Design review of the part built by this model. Coordinates are the model's own, in mm. A direction names the side the tool comes from. Round coordinates to 2 decimals unless told otherwise and drop trailing zeros. Loops run counter-clockwise (first coordinate to the right, second up) from the corner with the lowest first, then second, coordinate; pieces in that order, holes last. Notation, with made-up numbers: (59.25, 65.5) -> (93.25, 65.5) arc R22 ccw to (93.25, 84.5) -> close; hole circle Ø11 at (-40, -8). An arc over 180 degrees is marked (long way). Answer as CSV lines item,"result". Start each with the question number.
(1) Draft analysis for pull direction X (two halves, no side actions). For faces 4 (the face through (-19.15, -107.74, 0.64)), 5 (the face through (-75.61, 27.47, 0.63)), 6 (the face through (-34.96, -102.51, 0.63)), state which applies: +X half, -X half, draft (parallel to the pull), parting line (faces both ways), or undercut.
(2) Take a section at C-C, the plane y = -41. Write out the cut boundary in (x, z) (3 decimals), and give its area (3 significant figures).
(3) Take a section at D-D, the plane x = -88. Write out the cut boundary in (y, z), and give its area (3 significant figures).
(4) Take a section at A-A, the plane x = -77.55. Write out the cut boundary in (y, z).
(5) To check wall thickness, follow line 1 (Y direction, x = -87.55, z = 1); line 2 (Y direction, x = -77.55, z = 0.85); line 3 (X direction, y = -92.5, z = 0.2). State the ranges of each line that lie inside material, in increasing order. Write a range as from..to.
(6) Machinability: for faces 1 (the face through (-59.822, -63.878, 0.644)), 2 (the face through (-41.71, -87.56, 0.63)), 3 (the face through (-93.551, 30.795, 0.644)), which of the approach directions +Z, -Z, +X, -X, +Y, -Y give a long, thin tool a straight path to every point of the face, cutting with its end or side? Answer none if there is none.
(7) Take a section at B-B, the plane z = 0.3. State how many separate pieces and enclosed holes the cut face has, and give its area (3 significant figures).
(8) For P1, Ø4, axis at x = -87.55, y = 28.273, coming from the -Z side; P2, Ø6.5, axis at x = -87.55, y = -20.327, coming from the +Z side; P3, Ø0.6, axis at y = 11.5, z = 0.5, coming from the -X side, all flat-tipped, find the tip position at first contact; note any pin that passes through.
from build123d import *

# Parameters (mm, degrees)
SKETCH1_R                    = 2.099999991
BASE_FLANGE1_DEPTH           = 1.27
EDGE_FLANGE2_STRIP_W         = 6.5532
EDGE_FLANGE2_STRIP_H         = 1.27
EDGE_FLANGE2_STRIP_CUT_DEPTH = 59.775021713
EDGE_FLANGE2_DEPTH           = 59.775021713
SKETCH14_W                   = 1.779250061
SKETCH14_H                   = 41.153999988
CUT_EXTRUDE1_DEPTH           = 148.532360138
CUT_EXTRUDE_THIN2_START      = 2.868175785
CUT_EXTRUDE_THIN2_DEPTH      = 59.775021713
CUT_EXTRUDE_THIN2_START_2    = 9.218175785
CUT_EXTRUDE_THIN2_2_DEPTH    = 47.075021713
CUT_EXTRUDE_THIN2_3_DEPTH    = 59.775021713
CUT_EXTRUDE_THIN2_4_DEPTH    = 6.35
CUT_EXTRUDE_THIN2_START_3    = 56.293197498
CUT_EXTRUDE_THIN2_5_DEPTH    = 6.35
BOSS_EXTRUDE1_DEPTH          = 1.27
FILLET1_R                    = 25.4
FILLET2_R                    = 3.175


# Read off the part's stored shape, not the designer's step: Cut-Extrude-Thin2
# Sheet-metal steps are written as plain solids
with BuildPart() as part:
    # Sketch1 → Base-Flange1 (new body)
    with BuildSketch(Plane.XY):
        Polygon((-24.438645943, -113.029505435), (-19.05049227, -107.641351762), (-63.562879499, -63.128964533), (-66.675, -51.514372705), (-66.675, 31.75), (-94.45625, 31.75), (-94.45625, -51.514372705), (-80.565625, -65.404997705), (-68.951033172, -68.517118206), align=None)
        with Locations((-87.550000033, 28.272999969)):
            Circle(SKETCH1_R, mode=Mode.SUBTRACT)
        with Locations((-77.549999967, 28.272999969)):
            Circle(SKETCH1_R, mode=Mode.SUBTRACT)
        with Locations((-87.550000033, -20.327000113)):
            Circle(SKETCH1_R, mode=Mode.SUBTRACT)
        with Locations((-77.549999967, -20.327000113)):
            Circle(SKETCH1_R, mode=Mode.SUBTRACT)
        Polygon((-92.676999939, -16.604000066), (-83.05, -16.604000066), (-82.05, -16.604000066), (-72.423000061, -16.604000066), (-72.423000061, 24.549999922), (-82.05, 24.549999922), (-83.05, 24.549999922), (-92.676999939, 24.549999922), align=None, mode=Mode.SUBTRACT)
    extrude(amount=BASE_FLANGE1_DEPTH)

    # Edge-Flange2 strip (across the edge) → Edge-Flange2 strip cut (cut)
    with BuildSketch(Plane(origin=(-19.05049227, -107.641351762, 1.27), x_dir=(-0.707106781186551, -0.707106781186544, 3.4914813388431334e-15), z_dir=(-0.707106781186544, 0.707106781186551, 0))):
        with Locations((-1.27, -0.635)):
            Rectangle(EDGE_FLANGE2_STRIP_W, EDGE_FLANGE2_STRIP_H)
    extrude(amount=EDGE_FLANGE2_STRIP_CUT_DEPTH, mode=Mode.SUBTRACT)

    # Edge-Flange2 section (across the edge) → Edge-Flange2 (add)
    with BuildSketch(Plane(origin=(-19.05049227, -107.641351762, 1.27), x_dir=(-0.707106781186551, -0.707106781186544, 3.4914813388431334e-15), z_dir=(-0.707106781186544, 0.707106781186551, 0))):
        with BuildLine():
            Line((0, 0.7366), (0, 8.255))
            Line((0, 8.255), (1.27, 8.255))
            Line((1.27, 8.255), (1.27, 0.7366))
            ThreePointArc((1.27, 0.7366), (1.485745145, 0.215745145), (2.0066, 0))
            Line((2.0066, 0), (2.0066, -1.27))
            ThreePointArc((2.0066, -1.27), (0.587719533, -0.682280467), (0, 0.7366))
        make_face()
    extrude(amount=EDGE_FLANGE2_DEPTH)

    # Sketch14 → Cut-Extrude1 (cut, through all)
    with BuildSketch(Plane.XY.offset(1.27)):
        with Locations((-93.56662497, 3.972999928)):
            Rectangle(SKETCH14_W, SKETCH14_H)
    extrude(amount=-CUT_EXTRUDE1_DEPTH, mode=Mode.SUBTRACT)

    # Cut-Extrude-Thin2 outline → Cut-Extrude-Thin2 (cut)
    with BuildSketch(Plane(origin=(0, 0, 0), x_dir=(0.7071067811865438, 0.7071067811865512, 0), z_dir=(0.7071067811865511, -0.7071067811865441, 0)).offset(CUT_EXTRUDE_THIN2_START)):
        with BuildLine():
            Line((-91.591262036, 1.27), (-89.724750852, 1.27))
            ThreePointArc((-89.724750852, 1.27), (-89.619995324, 1.631698534), (-89.584662036, 2.0066))
            Line((-89.584662036, 2.0066), (-89.584662036, 9.525))
            Line((-89.584662036, 9.525), (-90.854662036, 9.525))
            Line((-90.854662036, 9.525), (-90.854662036, 2.0066))
            ThreePointArc((-90.854662036, 2.0066), (-91.070407181, 1.485745145), (-91.591262036, 1.27))
        make_face()
    extrude(amount=CUT_EXTRUDE_THIN2_DEPTH, mode=Mode.SUBTRACT)

    # Cut-Extrude-Thin2 2 outline → Cut-Extrude-Thin2 2 (cut)
    with BuildSketch(Plane(origin=(0, 0, 0), x_dir=(0.7071067811865438, 0.7071067811865512, 0), z_dir=(0.7071067811865511, -0.7071067811865441, 0)).offset(CUT_EXTRUDE_THIN2_START_2)):
        with BuildLine():
            ThreePointArc((-91.407505482, 0.008431566), (-90.480448103, 0.335511742), (-89.820005482, 1.063682305))
            Line((-89.820005482, 1.063682305), (-89.820005482, 1.27))
            Line((-89.820005482, 1.27), (-91.407505482, 1.27))
            Line((-91.407505482, 1.27), (-91.407505482, 0.008431566))
        make_face()
    extrude(amount=CUT_EXTRUDE_THIN2_2_DEPTH, mode=Mode.SUBTRACT)

    # Cut-Extrude-Thin2 3 outline → Cut-Extrude-Thin2 3 (add)
    with BuildSketch(Plane(origin=(0, 0, 0), x_dir=(0.7071067811865438, 0.7071067811865512, 0), z_dir=(0.7071067811865511, -0.7071067811865441, 0)).offset(CUT_EXTRUDE_THIN2_START)):
        with BuildLine():
            Line((-89.820005482, 0), (-82.117848928, 0))
            Line((-82.117848928, 0), (-82.117848928, 1.27))
            Line((-82.117848928, 1.27), (-89.724750852, 1.27))
            ThreePointArc((-89.724750852, 1.27), (-89.769455165, 1.165491634), (-89.820005482, 1.063682305))
            Line((-89.820005482, 1.063682305), (-89.820005482, 0))
        make_face()
        with BuildLine():
            Line((-91.591262036, 0), (-91.407505482, 0))
            Line((-91.407505482, 0), (-91.407505482, 0.008431566))
            ThreePointArc((-91.407505482, 0.008431566), (-91.49928709, 0.002109), (-91.591262036, 0))
        make_face()
    extrude(amount=CUT_EXTRUDE_THIN2_3_DEPTH)

    # Cut-Extrude-Thin2 4 outline → Cut-Extrude-Thin2 4 (add)
    with BuildSketch(Plane(origin=(0, 0, 0), x_dir=(0.7071067811865438, 0.7071067811865512, 0), z_dir=(0.7071067811865511, -0.7071067811865441, 0)).offset(CUT_EXTRUDE_THIN2_START)):
        with BuildLine():
            Line((-91.407505482, 0), (-89.820005482, 0))
            Line((-89.820005482, 0), (-89.820005482, 1.063682305))
            ThreePointArc((-89.820005482, 1.063682305), (-90.480448103, 0.335511742), (-91.407505482, 0.008431566))
            Line((-91.407505482, 0.008431566), (-91.407505482, 0))
        make_face()
    extrude(amount=CUT_EXTRUDE_THIN2_4_DEPTH)

    # Cut-Extrude-Thin2 5 outline → Cut-Extrude-Thin2 5 (add)
    with BuildSketch(Plane(origin=(0, 0, 0), x_dir=(0.7071067811865438, 0.7071067811865512, 0), z_dir=(0.7071067811865511, -0.7071067811865441, 0)).offset(CUT_EXTRUDE_THIN2_START_3)):
        with BuildLine():
            Line((-91.407505482, 0), (-89.820005482, 0))
            Line((-89.820005482, 0), (-89.820005482, 1.063682305))
            ThreePointArc((-89.820005482, 1.063682305), (-90.480448103, 0.335511742), (-91.407505482, 0.008431566))
            Line((-91.407505482, 0.008431566), (-91.407505482, 0))
        make_face()
    extrude(amount=CUT_EXTRUDE_THIN2_5_DEPTH)

    # Sketch17 → Boss-Extrude1 (add)
    with BuildSketch(Plane.XY.offset(1.27)):
        Polygon((-68.951033172, -68.517118206), (-80.565625, -65.404997705), (-60.360048728, -85.610573978), (-46.992008762, -90.476142615), align=None)
    extrude(amount=-BOSS_EXTRUDE1_DEPTH)

    # Fillet1
    fillet1_edges = [part.edges().sort_by_distance(p)[0] for p in [
        (-46.992008762, -90.476142615, 0.635),
    ]]
    fillet(fillet1_edges, radius=FILLET1_R)

    # Fillet2
    fillet2_edges = [part.edges().sort_by_distance(p)[0] for p in [
        (-94.45625, 31.75, 0.635),
        (-66.675, 31.75, 0.635),
        (-66.675, -51.514372705, 0.635),
        (-63.562879499, -63.128964533, 0.635),
        (-94.45625, -51.514372705, 0.635),
        (-24.438645943, -113.029505435, 0.635),
        (-60.360048728, -85.610573978, 0.635),
        (-13.770658087, -102.361517579, 0.635),
        (-56.037981286, -60.094194381, 0.635),
    ]]
    fillet(fillet2_edges, radius=FILLET2_R)


solid = part.part
The answers:
1,face 4,"+X half"
1,face 5,"undercut"
1,face 6,"-X half"
2,outline,"(-94.456, 0) -> (-66.675, 0) -> (-66.675, 1.27) -> (-94.456, 1.27) -> close"
2,area,"35.3 mm²"
3,outline,"(-57.97, 0) -> (-22.38, 0) -> (-22.38, 1.27) -> (-57.97, 1.27) -> close; (-18.28, 0) -> (-16.6, 0) -> (-16.6, 1.27) -> (-18.28, 1.27) -> close; (24.55, 0) -> (26.22, 0) -> (26.22, 1.27) -> (24.55, 1.27) -> close; (30.32, 0) -> (31.75, 0) -> (31.75, 1.27) -> (30.32, 1.27) -> close"
3,area,"51.3 mm²"
4,outline,"(-68.42, 0) -> (-22.43, 0) -> (-22.43, 1.27) -> (-68.42, 1.27) -> close; (-18.23, 0) -> (-16.6, 0) -> (-16.6, 1.27) -> (-18.23, 1.27) -> close; (24.55, 0) -> (26.17, 0) -> (26.17, 1.27) -> (24.55, 1.27) -> close; (30.37, 0) -> (31.75, 0) -> (31.75, 1.27) -> (30.37, 1.27) -> close"
5,line 1,"-58.42..-22.43, -18.23..-16.6, 24.55..26.17, 30.37..31.75"
5,line 2,"-68.42..-22.43, -18.23..-16.6, 24.55..26.17, 30.37..31.75"
5,line 3,"-45.21..-36.77, -34.52..-23.63"
6,face 1,"+Z, -Z, +Y"
6,face 2,"+Z, -Z"
6,face 3,"+Z, -Z, -X, +Y"
7,separate pieces,"1"
7,enclosed holes,"5"
7,area,"2,710 mm²"
8,P1,"through"
8,P2,"z = 1.27"
8,P3,"x = -72.42"
